from build123d import *

# Parameters (mm, degrees)
SKETCH1_W           = 2.4
SKETCH1_H           = 2.4
BOSS_EXTRUDE1_DEPTH = 8.35
SKETCH2_W           = 1.5
SKETCH2_H           = 1.5
CUT_EXTRUDE1_DEPTH  = 8
SKETCH3_W           = 0.4
SKETCH3_H           = 0.4
BOSS_EXTRUDE2_DEPTH = 3


with BuildPart() as part:
    # Sketch1 → Boss-Extrude1 (new body)
    with BuildSketch(Plane(origin=(0, 0, 0), x_dir=(1, 0, 0), z_dir=(0, 1, 0))):
        Rectangle(SKETCH1_W, SKETCH1_H)
    extrude(amount=BOSS_EXTRUDE1_DEPTH)

    # Sketch2 → Cut-Extrude1 (cut)
    with BuildSketch(Plane(origin=(0, 8.35, 0), x_dir=(1, 0, 0), z_dir=(0, 1, 0))):
        Rectangle(SKETCH2_W, SKETCH2_H)
    extrude(amount=-CUT_EXTRUDE1_DEPTH, mode=Mode.SUBTRACT)

    # Sketch3 → Boss-Extrude2 (add)
    with BuildSketch(Plane.XZ):
        Rectangle(SKETCH3_W, SKETCH3_H)
    extrude(amount=BOSS_EXTRUDE2_DEPTH)


solid = part.part
The listing builds one solid part. Answer for the finished solid, in the listing's coordinates (mm). A direction names the side the tool comes from. Give positions to 0.01 mm unless a question says otherwise; leave off trailing zeros. Loops run counter-clockwise (first coordinate to the right, second up) from the corner with the lowest first, then second, coordinate; pieces in that order, holes last. Notation, with made-up numbers: (77.25, -7) - (103.25, -7) arc R22 cw to (103.25, 19) - close; hole circle Ø5 at (64.25, 2.25). An arc over 180 degrees is marked (long way). Answer as a JSON object with one key per item and string values.
1. For a pull along X with two mould halves and no side action, classify faces 1 (the flat face through (0, 4, -1.2)), 2 (the flat face through (0.75, 4, 0)), 3 (the flat face through (1.2, 4, 0)), 4 (the flat face through (0, 4, 0.75)) as pulls with the +X half, pulls with the -X half, needs draft (parallel to the pull), parting line crosses it, or undercut.
Determined:
{"face 1": "needs draft", "face 2": "undercut", "face 3": "pulls with the +X half", "face 4": "undercut"}
2. A cutting plane is placed at B-B (x = 0). Write down the section's boundary in (y, z).
Determined:
{"outline": "(-3, -0.2) - (0, -0.2) - (0, -1.2) - (8.35, -1.2) - (8.35, -0.75) - (0.35, -0.75) - (0.35, 0.75) - (8.35, 0.75) - (8.35, 1.2) - (0, 1.2) - (0, 0.2) - (-3, 0.2) - close"}
3. A cutting plane is placed at A-A (y = 6). Write down the section's boundary in (x, z).
Determined:
{"outline": "(-1.2, -1.2) - (1.2, -1.2) - (1.2, 1.2) - (-1.2, 1.2) - close; hole (-0.75, -0.75) - (0.75, -0.75) - (0.75, 0.75) - (-0.75, 0.75) - close"}
4. A cutting plane is placed at C-C (z = 0.1). Write down the section's boundary in (x, y), then the cut area to 3 significant figures.
Determined:
{"outline": "(-1.2, 0) - (-0.2, 0) - (-0.2, -3) - (0.2, -3) - (0.2, 0) - (1.2, 0) - (1.2, 8.35) - (0.75, 8.35) - (0.75, 0.35) - (-0.75, 0.35) - (-0.75, 8.35) - (-1.2, 8.35) - close", "area": "9.24 mm²"}
5. Find the intervals of material crossed by L1, parallel to Z at x = 0.05, y = 4.5; L2, parallel to Y at x = -0.4, z = 0.05, in increasing order. Write a range as [from, to].
Determined:
{"L1": "[-1.2, -0.75], [0.75, 1.2]", "L2": "[0, 0.35]"}
6. For faces 5 (the flat face through (-0.75, 4, 0)), 6 (the flat face through (-1.2, 4, 0)), determine the directions among +Z, -Z, +X, -X, +Y, -Y from which every point of the face is accessible in a straight line to the end or side of a thin tool.
Determined:
{"face 5": "+Y", "face 6": "+Z, -Z, -X, +Y, -Y"}
7. A cutting plane is placed at D-D (y = -0.25). Write down the section's boundary in (x, z), then the cut area to 3 significant figures.
Determined:
{"outline": "(-0.2, -0.2) - (0.2, -0.2) - (0.2, 0.2) - (-0.2, 0.2) - close", "area": "0.160 mm²"}
